The model under review builds one solid part; all positions refer to its coordinate system, in mm. Face numbers are marked on the shaded views. A direction names the side the tool comes from. Give positions to 0.01 mm unless a question says otherwise; leave off trailing zeros. Loops run counter-clockwise (first coordinate to the right, second up) from the corner with the lowest first, then second, coordinate; pieces in that order, holes last. Notation, with made-up numbers: M -16,53 L 29,53 A13 ccw 29,64 Z; hole C 71.25,-17.5 d9. An arc over 180 degrees is marked long. Return JSON: item names as keys, results as strings.
```python
from build123d import *

# Parameters (mm, degrees)
F1_DEPTH = 6.25
F2_R     = 2.5
F3_DEPTH = 1
F4_R     = 2.5
F5_DEPTH = 1


with BuildPart() as f1:
    # F0 (on Top) → F1 (new body, symmetric)
    with BuildSketch(Plane.XY):
        with BuildLine():
            Line((-20, -14.5), (-20, 0))
            Line((-20, 0), (-21, 0))
            Line((-21, 0), (-21, -15.5))
            ThreePointArc((-21, -15.5), (-20.707107, -16.207107), (-20, -16.5))
            Line((-20, -16.5), (-2, -16.5))
            ThreePointArc((-2, -16.5), (-1.292893, -16.792893), (-1, -17.5))
            Line((-1, -17.5), (-1, -25.224715))
            ThreePointArc((-1, -25.224715), (-0.919371, -25.419371), (-0.724715, -25.5))
            Line((-0.724715, -25.5), (0, -25.5))
            Line((0, -25.5), (0, -16.5))
            ThreePointArc((0, -16.5), (-0.292893, -15.792893), (-1, -15.5))
            Line((-1, -15.5), (-19, -15.5))
            ThreePointArc((-19, -15.5), (-19.707107, -15.207107), (-20, -14.5))
        make_face()
        with BuildLine():
            Line((0, 16.5), (0, 25.5))
            Line((0, 25.5), (-0.724715, 25.5))
            ThreePointArc((-0.724715, 25.5), (-0.919371, 25.419371), (-1, 25.224715))
            Line((-1, 25.224715), (-1, 17.5))
            ThreePointArc((-1, 17.5), (-1.292893, 16.792893), (-2, 16.5))
            Line((-2, 16.5), (-20, 16.5))
            ThreePointArc((-20, 16.5), (-20.707107, 16.207107), (-21, 15.5))
            Line((-21, 15.5), (-21, 0))
            Line((-21, 0), (-20, 0))
            Line((-20, 0), (-20, 14.5))
            ThreePointArc((-20, 14.5), (-19.707107, 15.207107), (-19, 15.5))
            Line((-19, 15.5), (-1, 15.5))
            ThreePointArc((-1, 15.5), (-0.292893, 15.792893), (0, 16.5))
        make_face()
    extrude(amount=F1_DEPTH, both=True)

    # F2 (on face) → F3 (cut, through all)
    with BuildSketch(Plane.YZ):
        with BuildLine():
            Line((25.5, 6.25), (19.25, 6.25))
            ThreePointArc((19.25, 6.25), (23.669417, 4.419417), (25.5, 0))
            Line((25.5, 0), (25.5, 6.25))
        make_face()
        with Locations((20, 0)):
            Circle(F2_R)
        with BuildLine():
            Line((25.5, -6.25), (25.5, 0))
            ThreePointArc((25.5, 0), (23.669417, -4.419417), (19.25, -6.25))
            Line((19.25, -6.25), (25.5, -6.25))
        make_face()
        with Locations((-20, 0)):
            Circle(F2_R)
        with BuildLine():
            Line((-25.5, 6.25), (-25.5, 0))
            ThreePointArc((-25.5, 0), (-23.669417, 4.419417), (-19.25, 6.25))
            Line((-19.25, 6.25), (-25.5, 6.25))
        make_face()
        with BuildLine():
            Line((-25.5, -6.25), (-19.25, -6.25))
            ThreePointArc((-19.25, -6.25), (-23.669417, -4.419417), (-25.5, 0))
            Line((-25.5, 0), (-25.5, -6.25))
        make_face()
    extrude(amount=-F3_DEPTH, mode=Mode.SUBTRACT)

    # F4 (on face) → F5 (cut, through all)
    with BuildSketch(Plane(origin=(-21, 0, 0), x_dir=(0, -1, 0), z_dir=(-1, 0, 0))):
        Circle(F4_R)
    extrude(amount=-F5_DEPTH, mode=Mode.SUBTRACT)


solid = f1.part
```
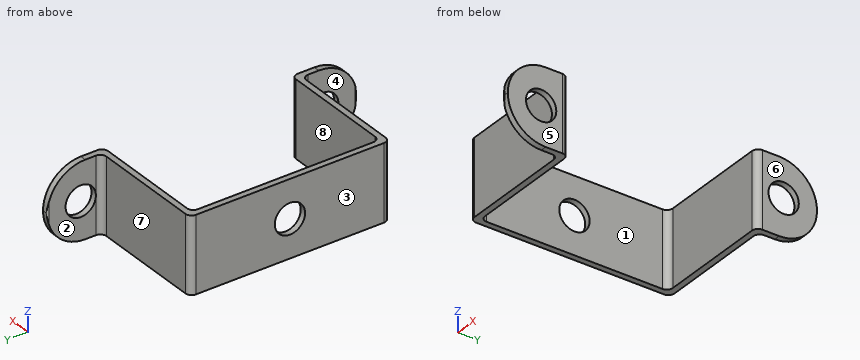
1) The part is to be moulded in two halves that separate along Y. For the marked faces 6, 7 and 8, say which applies: released by +Y, released by -Y, zero draft, split by the parting line, or undercut.
From the geometry:
{"face 6": "zero draft", "face 7": "released by +Y", "face 8": "undercut"}
2) Tool access review of the marked faces 1, 2, 3, 4 and 5: name each direction out of +Z, -Z, +X, -X, +Y, -Y from which nothing blocks a thin tool from reaching the whole face with its end or side.
From the geometry:
{"face 1": "+Z, -Z, +X", "face 2": "+Z, -Z, -X, +Y", "face 3": "+Z, -Z, -X, +Y, -Y", "face 4": "+Z, -Z, -X, -Y", "face 5": "+Z, -Z, +X, +Y, -Y"}
3) Consider section D-D on z = 5. Write out the cut boundary in (x, y), then the cut area to 3 significant figures.
From the geometry:
{"outline": "M -21,-15.5 A1 ccw -20,-16.5 L -2,-16.5 A1 cw -1,-17.5 L -1,-23 L 0,-23 L 0,-16.5 A1 ccw -1,-15.5 L -19,-15.5 A1 cw -20,-14.5 L -20,14.5 A1 cw -19,15.5 L -1,15.5 A1 ccw 0,16.5 L 0,23 L -1,23 L -1,17.5 A1 cw -2,16.5 L -20,16.5 A1 ccw -21,15.5 Z", "area": "86.0 mm²"}
4) Consider section A-A on x = -11.75. Write out the cut boundary in (y, z).
From the geometry:
{"outline": "M -16.5,-6.25 L -15.5,-6.25 L -15.5,6.25 L -16.5,6.25 Z; M 15.5,-6.25 L 16.5,-6.25 L 16.5,6.25 L 15.5,6.25 Z"}
5) Consider section B-B on y = 0. Write out the cut boundary in (x, z), then the cut area to 3 significant figures.
From the geometry:
{"outline": "M -21,-6.25 L -20,-6.25 L -20,-2.5 L -21,-2.5 Z; M -21,2.5 L -20,2.5 L -20,6.25 L -21,6.25 Z", "area": "7.50 mm²"}
6) Wall thickness on L1, parallel to Y at x = -12.5, z = 3.25; L2, parallel to X at y = -3.5, z = 1.5; L3, parallel to Z at x = -0.8, y = -20: over which ranges is each line inside the solid? List them lowest first. Write a range as from..to.
From the geometry:
{"L1": "-16.5..-15.5, 15.5..16.5", "L2": "-21..-20", "L3": "-6.2..-2.5, 2.5..6.2"}
7) Consider section C-C on z = -3.75. Write out the cut boundary in (x, y), then the cut area to 3 significant figures.
From the geometry:
{"outline": "M -21,-15.5 A1 ccw -20,-16.5 L -2,-16.5 A1 cw -1,-17.5 L -1,-24.25 L 0,-24.25 L 0,-16.5 A1 ccw -1,-15.5 L -19,-15.5 A1 cw -20,-14.5 L -20,14.5 A1 cw -19,15.5 L -1,15.5 A1 ccw 0,16.5 L 0,24.25 L -1,24.25 L -1,17.5 A1 cw -2,16.5 L -20,16.5 A1 ccw -21,15.5 Z", "area": "88.5 mm²"}
8) Insertion check: pin 1 (8 mm diameter, centred on x = -17.5, y = 2, fed in from -Z); pin 2 (6 mm diameter, centred on x = -8, z = 3, fed in from -Y); pin 3 (4 mm diameter, centred on x = -12, z = 2, fed in from +Y); pin 4 (2.5 mm diameter, centred on y = -20, z = -2, fed in from -X). Each pin has a flat end and moves straight along its axis. Give the tip position at first contact, or say it passes through.
From the geometry:
{"pin 1": "z = -6.25", "pin 2": "y = -16.5", "pin 3": "y = 16.5", "pin 4": "x = -1"}
